from build123d import *

# Parameters (mm, degrees)
SKETCH1_W           = 78
SKETCH1_H           = 126
SKETCH1_R           = 9
BOSS_EXTRUDE1_DEPTH = 13
SKETCH2_R           = 9
BOSS_EXTRUDE2_DEPTH = 13
BOSS_EXTRUDE3_DEPTH = 38
BOSS_EXTRUDE4_DEPTH = 51
BOSS_EXTRUDE5_DEPTH = 7.5
BOSS_EXTRUDE6_REACH = 100.539
SKETCH4_W           = 38
SKETCH4_H           = 15


with BuildPart() as part:
    # Sketch1 → Boss-Extrude1 (new body)
    with BuildSketch(Plane(origin=(0, 0, 0), x_dir=(1, 0, 0), z_dir=(0, 1, 0))):
        Rectangle(SKETCH1_W, SKETCH1_H)
        with Locations(Location((14, -44, 0), (0, 0, 90))):
            Circle(SKETCH1_R, mode=Mode.SUBTRACT)
        with Locations(Location((14, 44, 0), (0, 0, 90))):
            Circle(SKETCH1_R, mode=Mode.SUBTRACT)
    extrude(amount=BOSS_EXTRUDE1_DEPTH)

    # Sketch2 → Boss-Extrude2 (add)
    # profile 1 of 2: a face of its own
    with BuildSketch(Plane.ZY.offset(39)):
        with BuildLine():
            Line((0, 13), (63, 13))
            Line((63, 13), (63, 65))
            ThreePointArc((63, 65), (55.67766953, 82.67766953), (38, 90))
            Line((38, 90), (19.5, 90))
            Line((19.5, 90), (19.5, 66.644487847))
            ThreePointArc((19.5, 66.644487847), (23.58495283, 59.291561976), (25, 51))
            ThreePointArc((25, 51), (17.67766953, 33.32233047), (0, 26))
            Line((0, 26), (0, 13))
        make_face()
        with Locations((44, 65)):
            Circle(SKETCH2_R, mode=Mode.SUBTRACT)
    # profile 2 of 2: a face of its own
    with BuildSketch(Plane.ZY.offset(39)):
        with BuildLine():
            Line((-63, 13), (0, 13))
            Line((0, 13), (0, 26))
            ThreePointArc((0, 26), (-22.54009978, 40.18593962), (-19.5, 66.644487847))
            Line((-19.5, 66.644487847), (-19.5, 90))
            Line((-19.5, 90), (-38, 90))
            ThreePointArc((-38, 90), (-55.67766953, 82.67766953), (-63, 65))
            Line((-63, 65), (-63, 13))
        make_face()
        with Locations((-44, 65)):
            Circle(SKETCH2_R, mode=Mode.SUBTRACT)
    extrude(amount=-BOSS_EXTRUDE2_DEPTH)

    # Sketch2_3 → Boss-Extrude3 (add)
    with BuildSketch(Plane.ZY.offset(39)):
        with BuildLine():
            Line((-19.5, 90), (-19.5, 66.644487847))
            ThreePointArc((-19.5, 66.644487847), (-10.81406038, 73.54009978), (0, 76))
            Line((0, 76), (0, 80.5))
            ThreePointArc((0, 80.5), (-6.717514421, 83.282485579), (-9.5, 90))
            Line((-9.5, 90), (-19.5, 90))
        make_face()
        with BuildLine():
            Line((19.5, 66.644487847), (19.5, 90))
            Line((19.5, 90), (9.5, 90))
            ThreePointArc((9.5, 90), (6.717514421, 83.282485579), (0, 80.5))
            Line((0, 80.5), (0, 76))
            ThreePointArc((0, 76), (10.81406038, 73.54009978), (19.5, 66.644487847))
        make_face()
    extrude(amount=-BOSS_EXTRUDE3_DEPTH)

    # Sketch2_4 → Boss-Extrude4 (add)
    with BuildSketch(Plane.ZY.offset(39)):
        with BuildLine():
            ThreePointArc((-19.5, 66.644487847), (-22.54009978, 40.18593962), (0, 26))
            Line((0, 26), (0, 35))
            ThreePointArc((0, 35), (-16, 51), (0, 67))
            Line((0, 67), (0, 76))
            ThreePointArc((0, 76), (-10.81406038, 73.54009978), (-19.5, 66.644487847))
        make_face()
        with BuildLine():
            Line((0, 35), (0, 26))
            ThreePointArc((0, 26), (17.67766953, 33.32233047), (25, 51))
            ThreePointArc((25, 51), (23.58495283, 59.291561976), (19.5, 66.644487847))
            ThreePointArc((19.5, 66.644487847), (10.81406038, 73.54009978), (0, 76))
            Line((0, 76), (0, 67))
            ThreePointArc((0, 67), (11.313708499, 62.313708499), (16, 51))
            ThreePointArc((16, 51), (11.313708499, 39.686291501), (0, 35))
        make_face()
    extrude(amount=-BOSS_EXTRUDE4_DEPTH)

    # Sketch3 → Boss-Extrude5 (add, symmetric)
    with BuildSketch(Plane.XY):
        Polygon((-26, 13), (39, 13), (12, 25.03887683), (-26, 25.03887683), align=None)
    extrude(amount=BOSS_EXTRUDE5_DEPTH, both=True)

    # Sketch4 → Boss-Extrude6 (add, up to next)
    with BuildSketch(Plane(origin=(0, 25.03887683, 0), x_dir=(1, 0, 0), z_dir=(0, 1, 0)), mode=Mode.PRIVATE) as boss_extrude6_sk1:
        with Locations((-7, 0)):
            Rectangle(SKETCH4_W, SKETCH4_H)
    boss_extrude6_tool1 = extrude(boss_extrude6_sk1.sketch, amount=BOSS_EXTRUDE6_REACH, mode=Mode.PRIVATE) - part.part
    add(boss_extrude6_tool1.solids().sort_by_distance((-7, 25.038877, 0))[0])


solid = part.part
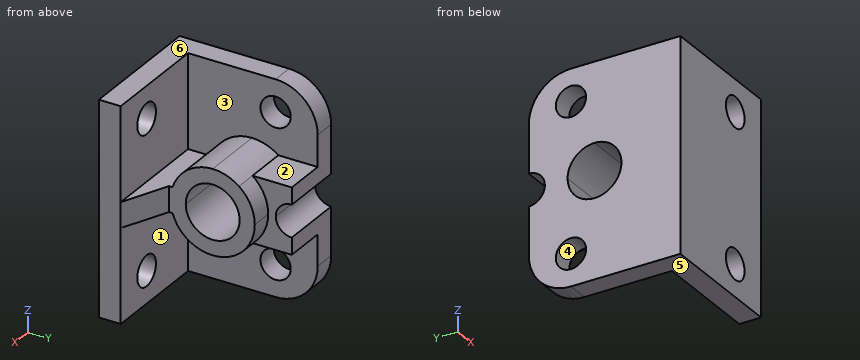
Input: part model. Units: mm. Frame: model coordinates. Face numbers are marked on the shaded views. A direction names the side the tool comes from. Give positions to 0.01 mm unless a question says otherwise; leave off trailing zeros. Write each loop counter-clockwise with the first axis right and the second up, starting at its lowest first coordinate (ties: lowest second). Pieces come first, ordered by that corner, then holes. Notation, with made-up numbers: (68.25, 67.5) -> (86.25, 67.5) arc R11 cw to (86.25, 72.5) -> close; hole circle Ø4 at (77.5, 29). An arc over 180 degrees is marked (long way). Use one line per item in the form item = value. Start each with the question number.
1) Ray query, probe 1 along X at (y, z) = (6.25, 44); probe 2 along Y at (x, z) = (9, -11.5); probe 3 along Z at (x, y) = (11, 9). Return the intervals inside material, ascending. Write a range as from..to.
2) Section query C-C on z = 51. Return the cut outline in (x, y).
3) Section query D-D on y = 70. Return the cut outline in (x, z), then the cut area to 3 significant figures.
4) Set-up query: the marked faces 1, 2 and 3. Return all of +Z, -Z, +X, -X, +Y, -Y with unobstructed straight access to the full face (end or side cutting, diameter ignored); none if empty.
5) Section query A-A on x = -4.5. Return the cut outline in (y, z).
6) Draft query along Z for the marked faces 4, 5 and 6. Return one class per face: pulls with the +Z half, pulls with the -Z half, needs draft (parallel to the pull), parting line crosses it, or undercut.
7) Pin query (flat end, axial travel): pin 1 (15.5 mm diameter, centred on x = 6.5, y = 23.5, fed in from -Z); pin 2 (16.5 mm diameter, centred on y = 64, z = 21.5, fed in from +X); pin 3 (7 mm diameter, centred on x = -13, y = 79.5, fed in from -Z); pin 4 (14.5 mm diameter, centred on y = 65, z = 44, fed in from +X). Return the tip coordinate at first contact, or that it passes through.
8) Section query B-B on y = 43. Return the cut outline in (x, z).
Outcome:
q1.probe_1 = -39..5, 23..39
q1.probe_2 = 0..13, 28.8..39.88, 62.12..73.2
q1.probe_3 = -63..-52.49, -35.51..35.51, 52.49..63
q2.outline = (-39, 0) -> (8.34, 0) -> (8.34, 13) -> (-26, 13) -> (-26, 59.34) -> (-39, 59.34) -> close; (-39, 70.66) -> (-26, 70.66) -> (-26, 86.35) -> (-39, 86.35) -> close; (19.66, 0) -> (39, 0) -> (39, 13) -> (19.66, 13) -> close
q3.outline = (-39, -62.49) -> (-26, -62.49) -> (-26, -51.48) -> (-39, -51.48) -> close; (-39, -36.52) -> (-26, -36.52) -> (-26, -19.5) -> (-1, -19.5) -> (-1, -16.25) -> (12, -16.25) -> (12, 16.25) -> (-1, 16.25) -> (-1, 19.5) -> (-26, 19.5) -> (-26, 36.52) -> (-39, 36.52) -> close; (-39, 51.48) -> (-26, 51.48) -> (-26, 62.49) -> (-39, 62.49) -> close
q3.area = 2,630 mm^2
q4.face_1 = -Z, +X
q4.face_2 = +Z, +X, +Y
q4.face_3 = +Z, +X
q5.outline = (0, -63) -> (13, -63) -> (13, -7.5) -> (27.15, -7.5) arc R25 ccw to (66.64, -19.5) -> (90, -19.5) -> (90, -9.5) arc R9.5 cw to (90, 9.5) -> (90, 19.5) -> (66.64, 19.5) arc R25 ccw to (27.15, 7.5) -> (13, 7.5) -> (13, 63) -> (0, 63) -> close; hole circle Ø32 at (51, 0)
q6.face_4 = undercut
q6.face_5 = pulls with the -Z half
q6.face_6 = pulls with the +Z half
q7.pin_1 = -15.33
q7.pin_2 = 12
q7.pin_3 = -19.5
q7.pin_4 = through
q8.outline = (-39, -63) -> (-26, -63) -> (-26, -23.69) -> (12, -23.69) -> (12, -13.86) -> (-39, -13.86) -> close; (-39, 13.86) -> (12, 13.86) -> (12, 23.69) -> (-26, 23.69) -> (-26, 63) -> (-39, 63) -> close
